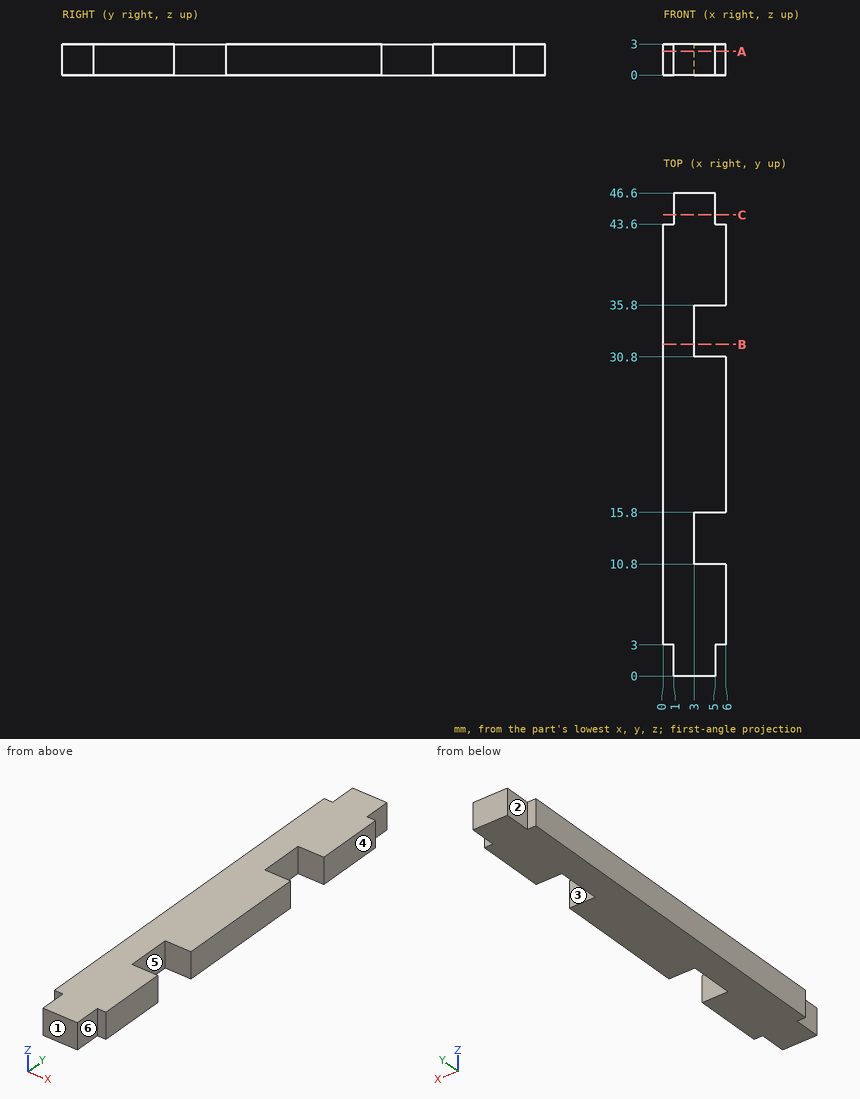
Answer from the drawing. Dimensions are ordinates in mm from the lowest x, y and z of the part. A direction names the side the tool comes from. Coordinates: 2 decimals unless noted, no trailing zeros. Write each loop counter-clockwise with the first axis right and the second up, starting at its lowest first coordinate (ties: lowest second). Pieces come first, ordered by that corner, then holes. Notation, with made-up numbers: (34.25, 31) - (47.25, 31) arc R12 cw to (47.25, 53) - close; hole circle Ø8 at (19, 79). An arc over 180 degrees is marked (long way). Return JSON: item names as keys, results as strings. Group by question number.
Q1. Which of the six approach directions +Z, -Z, +X, -X, +Y, -Y give full straight-line access (tool end or side, diameter ignored) to the marked faces 4, 5 and 6?
Q2. The part is cut by section A-A on z = 2.3. Write down the section's boundary in (x, y).
Q3. The part is cut by section B-B on y = 32. Write down the section's boundary in (x, z), and give its area (3 significant figures).
Q4. Find the intervals of material crossed by line 1 along Y through (x, z) = (5.4, 2.25); line 2 along Y through (x, z) = (4.65, 1.9); line 3 along X through (y, z) = (13.5, 0.3), in increasing order. Write a range as [from, to].
Q5. For a pull along Y with two mould halves and no side action, classify the marked faces 1, 2 and 3 as +Y half, -Y half, draft (parallel to the pull), parting line (faces both ways), or undercut.
Q6. Flat-ended cylindrical pins translate along their axes: pin 1 Ø0.9 at (y, z) = (45, 1) entering from -X; pin 2 Ø1.5 at (y, z) = (12.5, 1.5) entering from +X; pin 3 Ø1.5 at (y, z) = (45.5, 1.5) entering from +X. Find the tip coordinate at first contact, or state that the pin passes through.
Q7. The part is cut by section C-C on y = 44.5. Write down the section's boundary in (x, z), and give its area (3 significant figures).
Evaluation:
{
 "1": {"face 4": "+Z, -Z, +X, +Y, -Y", "face 5": "+Z, -Z, +X", "face 6": "+Z, -Z, +X, -Y"},
 "2": {"outline": "(0, 3) - (1, 3) - (1, 0) - (5, 0) - (5, 3) - (6, 3) - (6, 10.8) - (3, 10.8) - (3, 15.8) - (6, 15.8) - (6, 30.8) - (3, 30.8) - (3, 35.8) - (6, 35.8) - (6, 43.6) - (5, 43.6) - (5, 46.6) - (1, 46.6) - (1, 43.6) - (0, 43.6) - close"},
 "3": {"outline": "(0, 0) - (3, 0) - (3, 3) - (0, 3) - close", "area": "9.00 mm2"},
 "4": {"line 1": "y = [3, 10.8], [15.8, 30.8], [35.8, 43.6]", "line 2": "y = [0, 10.8], [15.8, 30.8], [35.8, 46.6]", "line 3": "x = [0, 3]"},
 "5": {"face 1": "-Y half", "face 2": "draft", "face 3": "undercut"},
 "6": {"pin 1": "stops at x = 1", "pin 2": "stops at x = 3", "pin 3": "stops at x = 5"},
 "7": {"outline": "(1, 0) - (5, 0) - (5, 3) - (1, 3) - close", "area": "12.0 mm2"}
}
